Design review of the part built by this model. Coordinates are the model's own, in mm. A direction names the side the tool comes from. Coordinates: 2 decimals unless noted, no trailing zeros. Loops run counter-clockwise (first coordinate to the right, second up) from the corner with the lowest first, then second, coordinate; pieces in that order, holes last. Notation, with made-up numbers: M 21.5,-25 L 35.5,-25 A26 ccw 35.5,0 Z; hole C -15.75,20 d11. An arc over 180 degrees is marked long. Answer as a JSON object with one key per item and string values. Group by question number.
1. To check wall thickness, follow probe 1 along X at (y, z) = (-1.4, 4.5); probe 2 along X at (y, z) = (-1, 9); probe 3 along Z at (x, y) = (-33.5, -1). State the ranges of each line that lie inside material, in increasing order.
2. Draft analysis for pull direction X (two halves, no side actions). For faces 1 (the cylindrical face through (-37.9, -1, 7.5)), 2 (the flat face through (-40.381, -0.986, 9.014)), 3 (the flat face through (-32.916, -1, 4)), state which applies: +X half, -X half, draft (parallel to the pull), parting line (faces both ways), or undercut.
3. Consider section B-B (y = -0.95). State the section outline as (x, z) points.
4. Consider section C-C (z = 6.75). State the section outline as (x, y) points, then the cut area to 3 significant figures.
5. Machinability: for faces 4 (the flat face through (-42.916, -1, 4)), 5 (the flat face through (-35.416, -1, 2)), which of the approach directions +Z, -Z, +X, -X, +Y, -Y give a long, thin tool a straight path to every point of the face, cutting with its end or side? Answer none if there is none.
6. Consider section A-A (z = 3.25). State the section outline as (x, y) points, then the cut area to 3 significant figures.
7. Consider section D-D (x = -41.75). State the section outline as (y, z) points, then the cut area to 3 significant figures.
from build123d import *

# Parameters (mm, degrees)
F1_DEPTH = 2
F3_DEPTH = 25


with BuildPart() as f1:
    # F0 (on Front) → F1 (new body)
    with BuildSketch(Plane.XZ):
        Polygon((-42.915918, 8), (-42.915918, 0), (-32.915918, 0), (-32.915918, 8), (-37.915918, 10), align=None)
    extrude(amount=F1_DEPTH)

    # F2 (on face) → F3 (cut)
    with BuildSketch(Plane.XZ.offset(2)):
        with BuildLine():
            ThreePointArc((-35.415918, 5), (-37.915918, 7.5), (-40.415918, 5))
            Line((-40.415918, 5), (-40.415918, 0))
            Line((-40.415918, 0), (-37.915918, 0))
            Line((-37.915918, 0), (-35.415918, 0))
            Line((-35.415918, 0), (-35.415918, 5))
        make_face()
    extrude(amount=-F3_DEPTH, mode=Mode.SUBTRACT)


solid = f1.part
Findings below:
{
 "1": {"probe 1": "x = -42.92 to -40.42, -35.42 to -32.92", "probe 2": "x = -40.42 to -35.42", "probe 3": "z = 0 to 8.23"},
 "2": {"face 1": "undercut", "face 2": "-X half", "face 3": "+X half"},
 "3": {"outline": "M -42.92,0 L -40.42,0 L -40.42,5 A2.5 cw -35.42,5 L -35.42,0 L -32.92,0 L -32.92,8 L -37.92,10 L -42.92,8 Z"},
 "4": {"outline": "M -42.92,-2 L -39.7,-2 L -39.7,0 L -42.92,0 Z; M -36.13,-2 L -32.92,-2 L -32.92,0 L -36.13,0 Z", "area": "12.9 mm^2"},
 "5": {"face 4": "+Z, -Z, -X, +Y, -Y", "face 5": "-Z, +Y, -Y"},
 "6": {"outline": "M -42.92,-2 L -40.42,-2 L -40.42,0 L -42.92,0 Z; M -35.42,-2 L -32.92,-2 L -32.92,0 L -35.42,0 Z", "area": "10.0 mm^2"},
 "7": {"outline": "M -2,0 L 0,0 L 0,8.47 L -2,8.47 Z", "area": "16.9 mm^2"}
}
